Verification items for the finished model (mm, model axes). Coordinates: 2 decimals unless noted, no trailing zeros. Order: outer loops, then holes, each group sorted by start corner. A loop starts at its lowest first (then second) coordinate and runs counter-clockwise, first axis right, second up. Notation, with made-up numbers: M -17,-1.75 L 5,-1.75 A16 ccw 5,9.25 Z; hole C 31.5,42 d8. An arc over 180 degrees is marked long. Return JSON: item names as keys, results as strings. Group by question number.
1. Material ranges on line 1 along Y through (x, z) = (-181.1, -0.5); line 2 along Y through (x, z) = (-113, 0.5); line 3 along Y through (x, z) = (-91.5, 2.5), recorded low to high.
2. Section check D-D, the plane x = -47. Record the cut outline in (y, z), plus the area to 3 significant figures.
3. Section check B-B, the plane z = 3. Give the number of separate pieces and of enclosed holes in the cut face, plus the area to 3 significant figures.
4. Section check C-C, the plane y = 36.5. Record the cut outline in (x, z).
5. Gauge pin test, flat ends, axial feed: pin 1 (4.5 mm diameter, centred on x = -157.5, z = 1.5, fed in from -Y); pin 2 (1.5 mm diameter, centred on x = -141.5, z = -3, fed in from +Y); pin 3 (1.5 mm diameter, centred on y = 8, z = 2.5, fed in from +X); pin 4 (5 mm diameter, centred on x = -181.1, y = 36.5, fed in from -Z). Record the tip position at first contact, or that the pin passes through.
6. Section check A-A, the plane x = -181.1. Record the cut outline in (y, z).
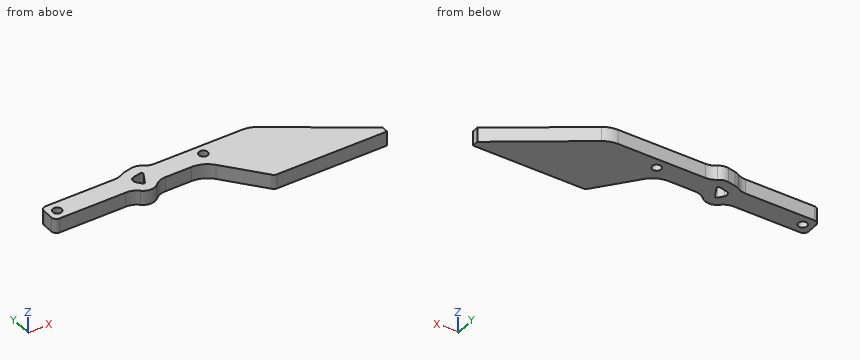
```python
from build123d import *

# Parameters (mm, degrees)
SKETCH3_R           = 2.75
BOSS_EXTRUDE3_DEPTH = 4.5
FILLET13_R          = 15
FILLET14_R          = 10
FILLET15_R          = 3


with BuildPart() as part:
    # Sketch3 → Boss-Extrude3 (new body, symmetric)
    with BuildSketch(Plane.XY):
        with BuildLine():
            Line((-70, 0), (0, 0))
            Line((0, 0), (0, 4))
            Line((0, 4), (-57, 43))
            Line((-57, 43), (-120.301993943, 43))
            ThreePointArc((-120.301993943, 43), (-123.692897096, 46.002238478), (-128.193883581, 46.505011528))
            Line((-128.193883581, 46.505011528), (-132.896667749, 45.573835187))
            ThreePointArc((-132.896667749, 45.573835187), (-135.482170861, 44.646108184), (-137.681223291, 43))
            Line((-137.681223291, 43), (-187, 43))
            Line((-187, 43), (-187, 30))
            Line((-187, 30), (-137.769349371, 30))
            Line((-137.769349371, 30), (-136.22697347, 27.997184072))
            ThreePointArc((-136.22697347, 27.997184072), (-129.680147263, 25.097686291), (-123.684421639, 29.011673389))
            Line((-123.684421639, 29.011673389), (-123.151115414, 30))
            Line((-123.151115414, 30), (-94.638255551, 30))
            Line((-94.638255551, 30), (-70, 0))
        make_face()
        with Locations((-90, 36.5)):
            Circle(SKETCH3_R, mode=Mode.SUBTRACT)
        with BuildLine():
            ThreePointArc((-133.278796519, 34.822100799), (-133.674163723, 37.467564533), (-131.634144466, 39.197626677))
            Line((-131.634144466, 39.197626677), (-126.931360298, 40.128803018))
            ThreePointArc((-126.931360298, 40.128803018), (-125.932483215, 39.741607136), (-125.857075346, 38.672967941))
            Line((-125.857075346, 38.672967941), (-129.404750544, 32.09839288))
            ThreePointArc((-129.404750544, 32.09839288), (-130.204180628, 31.576527934), (-131.077090788, 31.963127638))
            Line((-131.077090788, 31.963127638), (-133.278796519, 34.822100799))
        make_face(mode=Mode.SUBTRACT)
        with Locations((-181.1, 36.5)):
            Circle(SKETCH3_R, mode=Mode.SUBTRACT)
    extrude(amount=BOSS_EXTRUDE3_DEPTH, both=True)

    # Fillet13
    fillet13_edges = [part.edges().sort_by_distance(p)[0] for p in [
        (-57, 43, 0),
        (-94.638255551, 30, 0),
    ]]
    fillet(fillet13_edges, radius=FILLET13_R)

    # Fillet14
    fillet14_edges = [part.edges().sort_by_distance(p)[0] for p in [
        (-120.301993943, 43, 0),
        (-137.681223291, 43, 0),
        (-137.769349371, 30, 0),
        (-123.151115414, 30, 0),
    ]]
    fillet(fillet14_edges, radius=FILLET14_R)

    # Fillet15
    fillet15_edges = [part.edges().sort_by_distance(p)[0] for p in [
        (-70, 0, 0),
        (-187, 30, 0),
        (-187, 43, 0),
    ]]
    fillet(fillet15_edges, radius=FILLET15_R)


solid = part.part
```
Answers follow:
{
 "1": {"line 1": "30 to 33.75, 39.25 to 43", "line 2": "30 to 43", "line 3": "25.97 to 34.2, 38.8 to 43"},
 "2": {"outline": "M 0,-4.5 L 36.16,-4.5 L 36.16,4.5 L 0,4.5 Z", "area": "325 mm^2"},
 "3": {"separate pieces": "1", "enclosed holes": "3", "area": "3,800 mm^2"},
 "4": {"outline": "M -187,-4.5 L -183.85,-4.5 L -183.85,4.5 L -187,4.5 Z; M -178.35,-4.5 L -133.85,-4.5 L -133.85,4.5 L -178.35,4.5 Z; M -127.03,-4.5 L -92.75,-4.5 L -92.75,4.5 L -127.03,4.5 Z; M -87.25,-4.5 L -47.5,-4.5 L -47.5,4.5 L -87.25,4.5 Z"},
 "5": {"pin 1": "y = 30", "pin 2": "y = 43", "pin 3": "x = -4.75", "pin 4": "through"},
 "6": {"outline": "M 30,-4.5 L 33.75,-4.5 L 33.75,4.5 L 30,4.5 Z; M 39.25,-4.5 L 43,-4.5 L 43,4.5 L 39.25,4.5 Z"}
}
